from build123d import *

# Parameters (mm, degrees)
SKETCH_1_W          = 100
SKETCH_1_H          = 100
EXTRUDE_1_DEPTH     = 3
SKETCH_9_W          = 20
SKETCH_9_H          = 100
SKETCH_9_R          = 1.5
EXTRUDE_5_DEPTH     = 3
FILLET_1_R          = 20
EXTRUDE_6_DEPTH     = 7.1
CUT_EXTRUDE_5_DEPTH = 100
SKETCH_12_W         = 3.129471857
SKETCH_12_H         = 20
EXTRUDE_7_DEPTH     = 7.1
CUT_EXTRUDE_6_DEPTH = 100
SKETCH_14_W         = 103.339960755
SKETCH_14_H         = 14.24407727
CUT_EXTRUDE_7_DEPTH = 4
SKETCH_25_W         = 30
SKETCH_25_H         = 1.6
EXTRUDE_13_DEPTH    = 7
SKETCH_26_W         = 30
SKETCH_26_H         = 1.6
EXTRUDE_14_DEPTH    = 7
FILLET_7_R          = 10


with BuildPart() as part:
    # 草图1 → 凸台-拉伸1 (new body)
    with BuildSketch(Plane(origin=(0, 0, 0), x_dir=(1, 0, 0), z_dir=(0, 1, 0))):
        with Locations((50, -50)):
            Rectangle(SKETCH_1_W, SKETCH_1_H)
    extrude(amount=EXTRUDE_1_DEPTH)

    # 草图9 → 凸台-拉伸5 (add)
    # profile 1 of 2: a face of its own
    with BuildSketch(Plane.XZ):
        with Locations((110, 50)):
            Rectangle(SKETCH_9_W, SKETCH_9_H)
        with Locations(Location((110, 75, 0), (0, 0, 270))):
            Circle(SKETCH_9_R, mode=Mode.SUBTRACT)
        with Locations(Location((110, 25, 0), (0, 0, 270))):
            Circle(SKETCH_9_R, mode=Mode.SUBTRACT)
    # profile 2 of 2: a face of its own
    with BuildSketch(Plane.XZ):
        with Locations((-10, 50)):
            Rectangle(SKETCH_9_W, SKETCH_9_H)
        with Locations(Location((-10, 75, 0), (0, 0, 270))):
            Circle(SKETCH_9_R, mode=Mode.SUBTRACT)
        with Locations(Location((-10, 25, 0), (0, 0, 270))):
            Circle(SKETCH_9_R, mode=Mode.SUBTRACT)
    extrude(amount=-EXTRUDE_5_DEPTH)

    # 圆角1
    fillet_1_edges = [part.edges().sort_by_distance(p)[0] for p in [
        (120, 1.5, 100),
        (120, 1.5, 0),
        (-20, 1.5, 0),
        (-20, 1.5, 100),
    ]]
    fillet(fillet_1_edges, radius=FILLET_1_R)

    # 草图10 → 凸台-拉伸6 (add)
    with BuildSketch(Plane.XZ):
        Polygon((7, 50), (7, 0), (12, 0), (12, 100), (7, 100), align=None)
        Polygon((93, 50), (93, 0), (88, 0), (88, 100), (93, 100), align=None)
    extrude(amount=EXTRUDE_6_DEPTH)

    # 草图11 → 切除-拉伸5 (cut)
    with BuildSketch(Plane.XY.offset(100)):
        with BuildLine():
            Line((88, -4.6), (88, -7.1))
            Line((88, -7.1), (90.5, -7.1))
            ThreePointArc((90.5, -7.1), (88.732233047, -6.367766953), (88, -4.6))
        make_face()
        with BuildLine():
            ThreePointArc((93, -4.6), (92.267766953, -6.367766953), (90.5, -7.1))
            Line((90.5, -7.1), (93, -7.1))
            Line((93, -7.1), (93, -4.6))
        make_face()
        with BuildLine():
            ThreePointArc((12, -4.6), (11.267766953, -6.367766953), (9.5, -7.1))
            Line((9.5, -7.1), (12, -7.1))
            Line((12, -7.1), (12, -4.6))
        make_face()
        with BuildLine():
            ThreePointArc((9.5, -7.1), (7.732233047, -6.367766953), (7, -4.6))
            Line((7, -4.6), (7, -7.1))
            Line((7, -7.1), (9.5, -7.1))
        make_face()
    extrude(amount=-CUT_EXTRUDE_5_DEPTH, mode=Mode.SUBTRACT)

    # 草图12 → 凸台-拉伸7 (add)
    with BuildSketch(Plane.XZ):
        with Locations((98.435264072, 90)):
            Rectangle(SKETCH_12_W, SKETCH_12_H)
        with Locations((98.435264072, 10)):
            Rectangle(SKETCH_12_W, SKETCH_12_H)
    extrude(amount=EXTRUDE_7_DEPTH)

    # 草图13 → 切除-拉伸6 (cut)
    with BuildSketch(Plane(origin=(100, 0, 0), x_dir=(0, 0, -1), z_dir=(1, 0, 0))):
        with BuildLine():
            Line((-100, -7.1), (-100, 0))
            ThreePointArc((-100, 0), (-90.611432514, -5.27234511), (-80, -7.1))
            Line((-80, -7.1), (-100, -7.1))
        make_face()
        with BuildLine():
            Line((-20, -7.1), (0, -7.1))
            Line((0, -7.1), (0, 0))
            ThreePointArc((0, 0), (-9.388567486, -5.27234511), (-20, -7.1))
        make_face()
    extrude(amount=-CUT_EXTRUDE_6_DEPTH, mode=Mode.SUBTRACT)

    # 草图14 → 切除-拉伸7 (cut)
    with BuildSketch(Plane(origin=(100, 0, 0), x_dir=(0, 0, -1), z_dir=(1, 0, 0))):
        with Locations((-48.330019622, -7.122038635)):
            Rectangle(SKETCH_14_W, SKETCH_14_H)
    extrude(amount=-CUT_EXTRUDE_7_DEPTH, mode=Mode.SUBTRACT)

    # 草图25 → 凸台-拉伸13 (add)
    with BuildSketch(Plane.ZY.offset(-88)):
        with Locations((65, -3.8)):
            Rectangle(SKETCH_25_W, SKETCH_25_H)
        with Locations((35, -3.8)):
            Rectangle(SKETCH_25_W, SKETCH_25_H)
    extrude(amount=-EXTRUDE_13_DEPTH)

    # 草图26 → 凸台-拉伸14 (add)
    with BuildSketch(Plane(origin=(12, 0, 0), x_dir=(0, 0, -1), z_dir=(1, 0, 0))):
        with Locations((-65, -3.8)):
            Rectangle(SKETCH_26_W, SKETCH_26_H)
        with Locations((-35, -3.8)):
            Rectangle(SKETCH_26_W, SKETCH_26_H)
    extrude(amount=-EXTRUDE_14_DEPTH)

    # 圆角7
    # the kernel refuses this fillet: 10 mm, written as the material it takes off along each edge
    with BuildSketch(Plane(origin=(95, 12, 20), x_dir=(-1, 0, 0), z_dir=(0, -1, 0))) as fillet_7_piece_1_section:
        with BuildLine():
            CenterArc((10, -6), FILLET_7_R, 143.130102354, 36.869897646)
            Line((0, -6), (0, 0))
            Line((0, 0), (2, 0))
        make_face()
    fillet_7_piece_1 = extrude(amount=31.6, mode=Mode.PRIVATE)
    fillet_7_piece_1 = split(fillet_7_piece_1, bisect_by=Plane(origin=(94.505806646, 0, 22.831397785), z_dir=(0, -1, 0)), keep=Keep.TOP, mode=Mode.PRIVATE)
    add(fillet_7_piece_1, mode=Mode.SUBTRACT)
    with BuildSketch(Plane(origin=(95, -19.6, 80), x_dir=(0, 0, -1), z_dir=(0, 1, 0))) as fillet_7_piece_2_section:
        with BuildLine():
            CenterArc((6, 10), FILLET_7_R, 233.130102354, 36.869897646)
            Line((0, 2), (0, 0))
            Line((0, 0), (6, 0))
        make_face()
    fillet_7_piece_2 = extrude(amount=31.6, mode=Mode.PRIVATE)
    fillet_7_piece_2 = split(fillet_7_piece_2, bisect_by=Plane(origin=(94.505806646, 0, 77.168602215), z_dir=(0, -1, 0)), keep=Keep.TOP, mode=Mode.PRIVATE)
    add(fillet_7_piece_2, mode=Mode.SUBTRACT)
    with BuildSketch(Plane(origin=(5, -19.6, 20), x_dir=(0, 0, 1), z_dir=(0, 1, 0))) as fillet_7_piece_3_section:
        with BuildLine():
            CenterArc((6, 10), FILLET_7_R, 233.130102354, 36.869897646)
            Line((0, 2), (0, 0))
            Line((0, 0), (6, 0))
        make_face()
    fillet_7_piece_3 = extrude(amount=31.6, mode=Mode.PRIVATE)
    fillet_7_piece_3 = split(fillet_7_piece_3, bisect_by=Plane(origin=(5.494193354, 0, 22.831397785), z_dir=(0, -1, 0)), keep=Keep.TOP, mode=Mode.PRIVATE)
    add(fillet_7_piece_3, mode=Mode.SUBTRACT)
    with BuildSketch(Plane(origin=(5, 12, 80), x_dir=(1, 0, 0), z_dir=(0, -1, 0))) as fillet_7_piece_4_section:
        with BuildLine():
            CenterArc((10, -6), FILLET_7_R, 143.130102354, 36.869897646)
            Line((0, -6), (0, 0))
            Line((0, 0), (2, 0))
        make_face()
    fillet_7_piece_4 = extrude(amount=31.6, mode=Mode.PRIVATE)
    fillet_7_piece_4 = split(fillet_7_piece_4, bisect_by=Plane(origin=(5.494193354, 0, 77.168602215), z_dir=(0, -1, 0)), keep=Keep.TOP, mode=Mode.PRIVATE)
    add(fillet_7_piece_4, mode=Mode.SUBTRACT)


solid = part.part
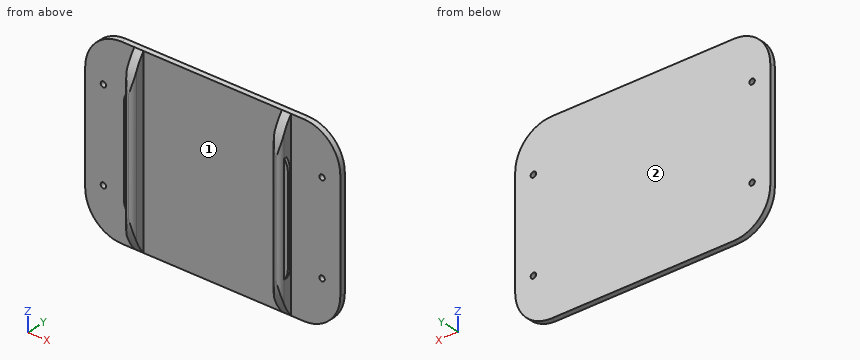
Source: CAD feature listing. Evaluate the final solid. Frame: model axes, mm. Face numbers are marked on the shaded views. Round coordinates to 2 decimals unless told otherwise and drop trailing zeros. Loops run counter-clockwise (first coordinate to the right, second up) from the corner with the lowest first, then second, coordinate; pieces in that order, holes last. Notation, with made-up numbers: (64, 11.5) - (73, 11.5) arc R19 ccw to (73, 46.5) - close; hole circle Ø2 at (-12.5, -32). An arc over 180 degrees is marked (long way). Write item = value, one per line. Start each with the question number.
Item 1: Section query C-C on x = 71.5. Output: boundary loops of the cut face in (y, z).
Item 2: Section query D-D on z = 84.5. Output: boundary loops of the cut face in (x, y), plus the area to 3 significant figures.
Item 3: First-contact query: pin 1 Ø2.5 at (y, z) = (-2, 49.5) entering from -X; pin 2 Ø8 at (x, z) = (112.5, 38) entering from -Y; pin 3 Ø1.4 at (y, z) = (-2.5, 65.5) entering from +X; pin 4 Ø4 at (x, y) = (17.5, -1) entering from +Z. Flat tips, straight axial feed; report the tip coordinate or a pass-through.
Item 4: Section query A-A on z = 32.5. Output: boundary loops of the cut face in (x, y).
Item 5: Mould query, pull axis X, two halves, no side actions, for the marked faces 1 and 2. Classes: released by +X, released by -X, zero draft, split by the parting line, or undercut.
Item 6: Section query B-B on x = -10. Output: boundary loops of the cut face in (y, z), plus the area to 3 significant figures.
Item 7: Material intervals for line 1 (X direction, y = 0.9, z = 75); line 2 (X direction, y = -4.5, z = 67); line 3 (Z direction, x = 110, y = 1.65), sorted ascending.
Results list:
q1.outline = (0, 0) - (3, 0) - (3, 100) - (0, 100) - close
q2.outline = (-19.49, 0) - (7, 0) - (7, -4.6) arc R2.5 ccw to (8.27, -6.78) - (10.73, -6.78) arc R2.5 ccw to (12, -4.6) - (12, 0) - (88, 0) - (88, -4.6) arc R2.5 ccw to (89.27, -6.78) - (91.73, -6.78) arc R2.5 ccw to (93, -4.6) - (93, 0) - (119.49, 0) - (119.49, 3) - (-19.49, 3) - close
q2.area = 481 mm²
q3.pin_1 = 5
q3.pin_2 = 0
q3.pin_3 = 95
q3.pin_4 = 100
q4.outline = (-20, 0) - (7, 0) - (7, -3) - (5, -3) - (5, -4.6) - (7, -4.6) arc R2.5 ccw to (12, -4.6) - (12, 0) - (88, 0) - (88, -4.6) arc R2.5 ccw to (93, -4.6) - (95, -4.6) - (95, -3) - (93, -3) - (93, 0) - (120, 0) - (120, 3) - (-20, 3) - close
q5.face_1 = undercut
q5.face_2 = zero draft
q6.outline = (0, 2.68) - (3, 2.68) - (3, 23.5) - (0, 23.5) - close; (0, 26.5) - (3, 26.5) - (3, 73.5) - (0, 73.5) - close; (0, 76.5) - (3, 76.5) - (3, 97.32) - (0, 97.32) - close
q6.area = 266 mm²
q7.line_1 = -20 to -11.5, -8.5 to 108.5, 111.5 to 120
q7.line_2 = 5 to 12, 88 to 95
q7.line_3 = 2.68 to 23.5, 26.5 to 73.5, 76.5 to 97.32
